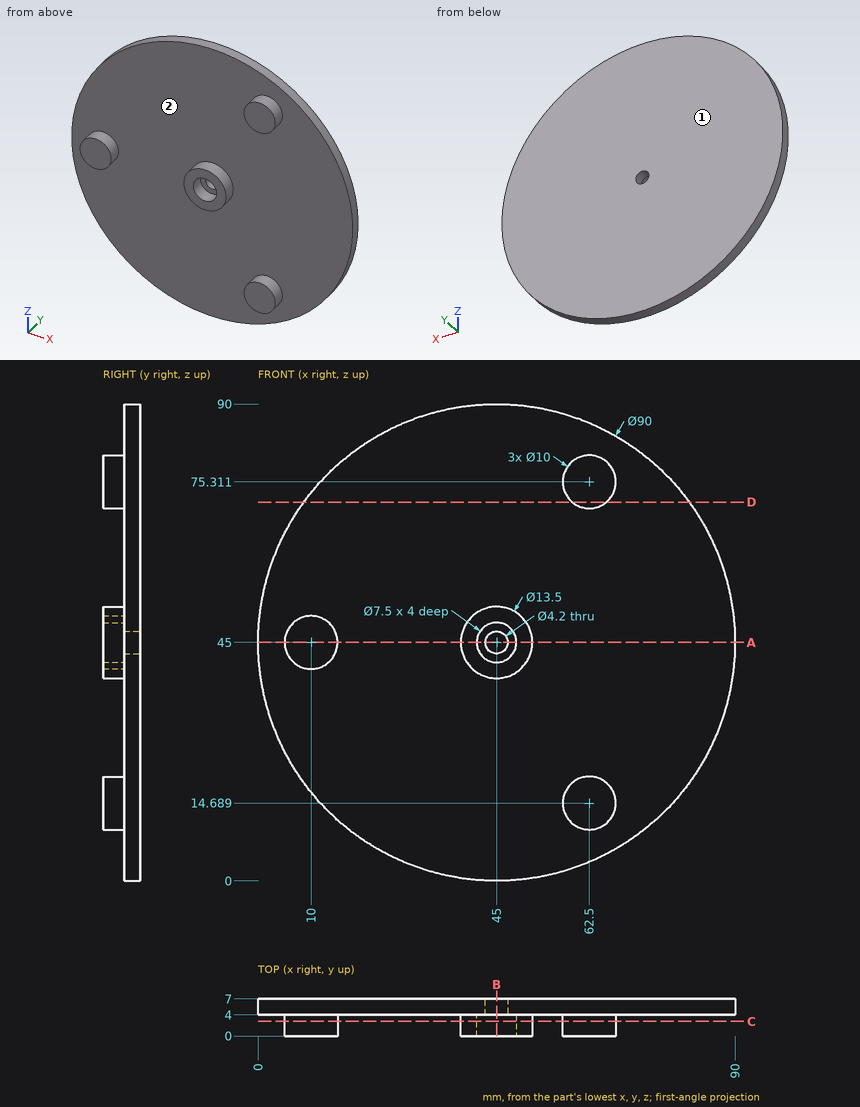
Can you work these out from the drawing? Everything is in mm from the part's minimum corner. A direction names the side the tool comes from. Coordinates: 2 decimals unless noted, no trailing zeros. Write each loop counter-clockwise with the first axis right and the second up, starting at its lowest first coordinate (ties: lowest second). Pieces come first, ordered by that corner, then holes. Notation, with made-up numbers: (84.5, 81) -> (120.5, 81) arc R16 ccw to (120.5, 111) -> close; hole circle Ø9 at (-25.5, 58.25). An arc over 180 degrees is marked (long way). Write item = value, one per line.
(1) Imagine slicing it at C-C (y = 2.75). Please give me the cut outline in (x, z), and give its area (3 significant figures).
Verdict:
outline = circle Ø10 at (10, 45); circle Ø13.5 at (45, 45); circle Ø10 at (62.5, 14.69); circle Ø10 at (62.5, 75.31); hole circle Ø7.5 at (45, 45)
area = 335 mm^2
(2) Imagine slicing it at D-D (z = 71.5). Please give me the cut outline in (x, y), and give its area (3 significant figures).
Verdict:
outline = (8.63, 4) -> (59.26, 4) -> (59.26, 0) -> (65.74, 0) -> (65.74, 4) -> (81.37, 4) -> (81.37, 7) -> (8.63, 7) -> close
area = 244 mm^2
(3) If I drill on probe 1 along X at (y, z) = (6.45, 45); probe 2 along Z at (x, y) = (45, 2.05), over which ranges is the centre line in solid material (lowest first)?
Verdict:
probe_1 = 0 to 42.9, 47.1 to 90
probe_2 = 38.25 to 41.25, 48.75 to 51.75
(4) On a 3-axis mill with a long thin cutter (end or side, diameter ignored), from which of +Z, -Z, +X, -X, +Y, -Y can I reach the whole of each face in a straight line? I mean the marked faces 1 and 2. Say none if no direction works.
Verdict:
face_1 = +Z, -Z, +X, -X, +Y
face_2 = -Y
(5) For pin 1 (3.5 mm diameter, centred on x = 45, z = 45, fed in from +Y); pin 2 (1 mm diameter, centred on x = 72.5, z = 37, fed in from -Y); pin 3 (4 mm diameter, centred on y = 4.5, z = 18.5, fed in from -X); pin 4 (1 mm diameter, centred on x = 41.5, y = 5.5, fed in from +Z), each with a flat end and sliding along its axis, tell me the tip position at first contact or that it passes through.
Verdict:
pin_1 = through
pin_2 = 4
pin_3 = 7.25
pin_4 = 89.9
(6) Imagine slicing it at B-B (x = 45). Please give me the cut outline in (y, z).
Verdict:
outline = (0, 38.25) -> (4, 38.25) -> (4, 0) -> (7, 0) -> (7, 42.9) -> (4, 42.9) -> (4, 41.25) -> (0, 41.25) -> close; (0, 48.75) -> (4, 48.75) -> (4, 47.1) -> (7, 47.1) -> (7, 90) -> (4, 90) -> (4, 51.75) -> (0, 51.75) -> close
(7) Imagine slicing it at A-A (z = 45). Please give me the cut outline in (x, y).
Verdict:
outline = (0, 4) -> (5, 4) -> (5, 0) -> (15, 0) -> (15, 4) -> (38.25, 4) -> (38.25, 0) -> (41.25, 0) -> (41.25, 4) -> (42.9, 4) -> (42.9, 7) -> (0, 7) -> close; (47.1, 4) -> (48.75, 4) -> (48.75, 0) -> (51.75, 0) -> (51.75, 4) -> (90, 4) -> (90, 7) -> (47.1, 7) -> close
